The model under review builds one solid part; all positions refer to its coordinate system, in mm. Round coordinates to 2 decimals unless told otherwise and drop trailing zeros. Write each loop counter-clockwise with the first axis right and the second up, starting at its lowest first coordinate (ties: lowest second). Pieces come first, ordered by that corner, then holes.
Item 1: To check wall thickness, follow L1, parallel to X at y = 12, z = -5.5; L2, parallel to Z at x = 3, y = 12; L3, parallel to X at y = 7.5, z = -38. State the ranges of each line that lie inside material, in increasing order.
Item 2: Add section D-D (y = 9). Give the boundary of the cut face in (x, z), plus the area to 3 significant figures.
Item 3: Add section A-A (x = 8). Give the boundary of the cut face in (y, z), plus the area to 3 significant figures.
Item 4: Clearance check with a flat-ended pin moving along its axis: pin 1 Ø1.5 at (y, z) = (2, -60) entering from -X. State where the tip first meets the part, or that it passes through.
Item 5: Add section C-C (z = -5). Give the boundary of the cut face in (x, y), plus the area to 3 significant figures.
```python
from build123d import *

# Parameters (mm, degrees)
SKETCH1_W           = 76.2
SKETCH1_H           = 76.2
BOSS_EXTRUDE1_DEPTH = 12.7
SKETCH2_W           = 25.4
SKETCH2_H           = 10.414
SKETCH2_W_2         = 10.414
SKETCH2_H_2         = 25.4
CUT_EXTRUDE1_DEPTH  = 6.35
SKETCH3_W           = 76.2
SKETCH3_H           = 76.2
BOSS_EXTRUDE2_DEPTH = 0.0254


with BuildPart() as part:
    # Sketch1 → Boss-Extrude1 (new body)
    with BuildSketch(Plane(origin=(0, 0, 0), x_dir=(1, 0, 0), z_dir=(0, 1, 0))):
        with Locations((38.1, 38.1)):
            Rectangle(SKETCH1_W, SKETCH1_H)
    extrude(amount=BOSS_EXTRUDE1_DEPTH)

    # Sketch2 → Cut-Extrude1 (cut)
    with BuildSketch(Plane(origin=(0, 12.7, 0), x_dir=(1, 0, 0), z_dir=(0, 1, 0))):
        with Locations((38.1, 70.993)):
            Rectangle(SKETCH2_W, SKETCH2_H)
        with Locations((5.207, 38.1)):
            Rectangle(SKETCH2_W_2, SKETCH2_H_2)
        with Locations((38.1, 5.207)):
            Rectangle(SKETCH2_W, SKETCH2_H)
        with Locations((70.993, 38.1)):
            Rectangle(SKETCH2_W_2, SKETCH2_H_2)
    extrude(amount=-CUT_EXTRUDE1_DEPTH, mode=Mode.SUBTRACT)

    # Sketch3 → Boss-Extrude2 (add)
    with BuildSketch(Plane(origin=(0, 12.7, 0), x_dir=(1, 0, 0), z_dir=(0, 1, 0))):
        with Locations((38.1, 38.1)):
            Rectangle(SKETCH3_W, SKETCH3_H)
    extrude(amount=BOSS_EXTRUDE2_DEPTH)


solid = part.part
```
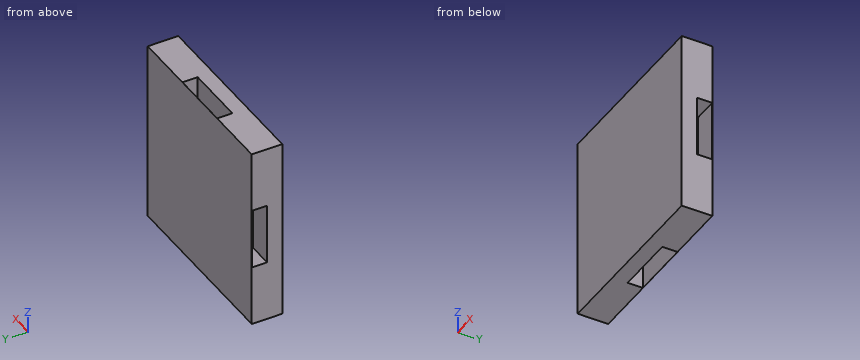
Numbers:
1. L1: x = 0 to 25.4, 50.8 to 76.2
1. L2: z = -76.2 to -50.8, -25.4 to 0
1. L3: x = 10.41 to 65.79
2. outline: (0, -76.2) - (25.4, -76.2) - (25.4, -65.79) - (50.8, -65.79) - (50.8, -76.2) - (76.2, -76.2) - (76.2, -50.8) - (65.79, -50.8) - (65.79, -25.4) - (76.2, -25.4) - (76.2, 0) - (50.8, 0) - (50.8, -10.41) - (25.4, -10.41) - (25.4, 0) - (0, 0) - (0, -25.4) - (10.41, -25.4) - (10.41, -50.8) - (0, -50.8) - close
2. area: 4,750 mm2
3. outline: (0, -76.2) - (12.73, -76.2) - (12.73, 0) - (0, 0) - close; hole (6.35, -50.8) - (12.7, -50.8) - (12.7, -25.4) - (6.35, -25.4) - close
3. area: 808 mm2
4. pin 1: stops at x = 0
5. outline: (0, 0) - (76.2, 0) - (76.2, 12.73) - (0, 12.73) - close; hole (25.4, 6.35) - (50.8, 6.35) - (50.8, 12.7) - (25.4, 12.7) - close
5. area: 808 mm2
